```python
from build123d import *

# Parameters (mm, degrees)
F1_DEPTH = 200
F2_R     = 5
F3_DEPTH = 5
F4_R     = 5


with BuildPart() as f1:
    # F0 (on Top) → F1 (new body)
    with BuildSketch(Plane.XY):
        with BuildLine():
            ThreePointArc((-5, -25.0049995001), (0, 25.5), (5, -25.0049995001))
            Line((5, -25.0049995001), (5, -35.1461235416))
            ThreePointArc((5, -35.1461235416), (26.8118443976, -23.2674665574), (35.5, 0))
            Line((35.5, 0), (35.5, 35.5))
            Line((35.5, 35.5), (0, 35.5))
            Line((0, 35.5), (-35.5, 35.5))
            Line((-35.5, 35.5), (-35.5, 0))
            ThreePointArc((-35.5, 0), (-26.8118443976, -23.2674665574), (-5, -35.1461235416))
            Line((-5, -35.1461235416), (-5, -25.0049995001))
        make_face()
    extrude(amount=F1_DEPTH)

    # F2
    f2_edges = [f1.edges().sort_by_distance(p)[0] for p in [
        (-5, -35.146124, 100),
        (5, -35.146124, 100),
    ]]
    fillet(f2_edges, radius=F2_R)

    # F3 (add): a face of the model
    f3_faces = [f1.faces().sort_by_distance(p)[0] for p in [
        (0, 35.5, 100),
    ]]
    extrude(f3_faces, amount=F3_DEPTH)

    # F4
    f4_edges = [f1.edges().sort_by_distance(p)[0] for p in [
        (35.5, 40.5, 100),
        (-35.5, 40.5, 100),
    ]]
    fillet(f4_edges, radius=F4_R)


solid = f1.part
```
Part model, mm, in its own coordinate system. A direction names the side the tool comes from. Round coordinates to 2 decimals unless told otherwise and drop trailing zeros. Write each loop counter-clockwise with the first axis right and the second up, starting at its lowest first coordinate (ties: lowest second). Pieces come first, ordered by that corner, then holes. Notation, with made-up numbers: M 71,66.25 L 112,66.25 A23 cw 112,77.25 Z; hole C 33.25,89.25 d5. An arc over 180 degrees is marked long. Answer as CSV lines item,"result". Start each with the question number.
1) Band-saw the part on C-C (x = 0). List the corners of the cut face in (y, z).
2) Drop flat-ended pins along their axis: pin 1 (3 mm diameter, centred on y = -27, z = 62.5, fed in from +X); pin 2 (3 mm diameter, centred on x = 0, y = 22.5, fed in from -Z); pin 3 (4 mm diameter, centred on y = -26.5, z = 122, fed in from -X); pin 4 (10 mm diameter, centred on x = -9, z = 160.5, fed in from -Y). Give the stop position or say it passes through.
3) Band-saw the part on A-A (y = -18). List the corners of the cut face in (x, z), then the cut area to 3 significant figures.
4) Which spindle directions (+Z, -Z, +X, -X, +Y, -Y) get a long thin tool onto all of the face, cutting with end or side? Do faces 5 (the face through (-5, -27, 99)), 6 (the face through (-34.07, 39, 101.4)). Say none if no direction does.
5) Drill centre lines: L1, parallel to X at y = 0, z = 77.5; L2, parallel to Y at x = 0, z = 41.5; L3, parallel to Y at x = 13, z = 107. Where is each one in solid material? Low to high.
6) Mould opens along Y. For faces 1 (the face through (-1.05, 25.48, 98.6)), 2 (the face through (-35.5, 18, 99)), 3 (the face through (0, 40.5, 99)), 4 (the face through (-29.1, -20.33, 98.6)) say: +Y half, -Y half, draft (parallel to the pull), parting line (faces both ways), or undercut.
7) Band-saw the part on D-D (x = 28). List the corners of the cut face in (y, z), then the cut area to 3 significant figures.
8) Band-saw the part on B-B (z = 174). List the corners of the cut face in (x, y) (3 decimals).
Worked out:
1,outline,"M 25.5,0 L 40.5,0 L 40.5,200 L 25.5,200 Z"
2,pin 1,"x = 24.7"
2,pin 2,"through"
2,pin 3,"x = -25.69"
2,pin 4,"y = -33.81"
3,outline,"M -30.6,0 L -18.06,0 L -18.06,200 L -30.6,200 Z; M 18.06,0 L 30.6,0 L 30.6,200 L 18.06,200 Z"
3,area,"5,010 mm²"
4,face 5,"+Z, -Z, -Y"
4,face 6,"+Z, -Z, -X, +Y"
5,L1,"-35.5 to -25.5, 25.5 to 35.5"
5,L2,"25.5 to 40.5"
5,L3,"-33.03 to -21.94, 21.94 to 40.5"
6,face 1,"undercut"
6,face 2,"draft"
6,face 3,"+Y half"
6,face 4,"-Y half"
7,outline,"M -21.82,0 L 40.5,0 L 40.5,200 L -21.82,200 Z"
7,area,"12,500 mm²"
8,outline,"M -35.5,0 A35.5 ccw -11.639,-33.538 A5 ccw -5,-28.814 L -5,-25.005 A25.5 cw long 5,-25.005 L 5,-28.814 A5 ccw 11.639,-33.538 A35.5 ccw 35.5,0 L 35.5,35.5 A5 ccw 30.5,40.5 L -30.5,40.5 A5 ccw -35.5,35.5 Z"
